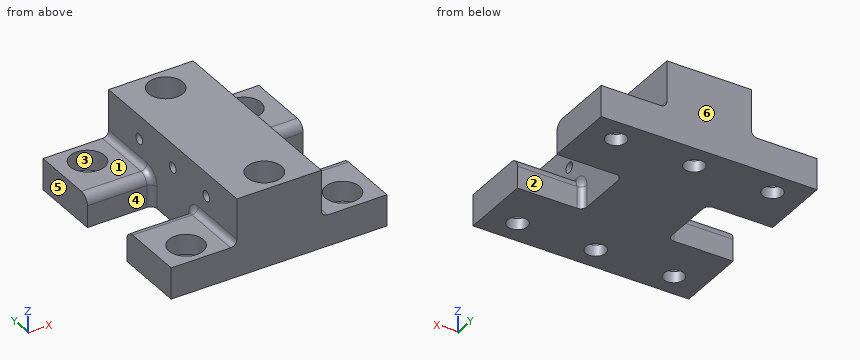
```python
from build123d import *

# Parameters (mm, degrees)
SKETCH_1_W                  = 69
SKETCH_1_H                  = 65
EXTRUDE_1_DEPTH             = 10
SKETCH_2_W                  = 27
SKETCH_2_H                  = 65
EXTRUDE_2_DEPTH             = 15
SKETCH_3_W                  = 10
SKETCH_3_H                  = 20
CUT_EXTRUDE_1_DEPTH         = 22
FILLET_1_R                  = 3
FILLET_2_R                  = 2
PATTERN_LINEAR_2_COUNT      = 2
PATTERN_LINEAR_2_PITCH      = 17
PATTERN_LINEAR_2_COL_COUNT  = 2
PATTERN_LINEAR_2_COL_PITCH  = 17
HOLE_WIZARD_M6_1_AT_2_COUNT = 2
HOLE_WIZARD_M6_1_AT_2_PITCH = 50
HOLE_WIZARD_M6_1_AT_3_COUNT = 2
HOLE_WIZARD_M6_1_AT_3_PITCH = 70.710678119
HOLE_WIZARD_M6_1_AT_4_COUNT = 2
HOLE_WIZARD_M6_1_AT_4_PITCH = 50
HOLE_WIZARD_M6_1_AT_5_COUNT = 2
HOLE_WIZARD_M6_1_AT_5_PITCH = 25
HOLE_WIZARD_M6_1_AT_6_COUNT = 2
HOLE_WIZARD_M6_1_AT_6_PITCH = 55.901699437
SKETCH_15_R                 = 5.5
CUT_EXTRUDE_3_DEPTH         = 16


with BuildPart() as part:
    # 스케치1 → 보스-돌출1 (new body)
    with BuildSketch(Plane.XY):
        Rectangle(SKETCH_1_W, SKETCH_1_H)
    extrude(amount=EXTRUDE_1_DEPTH)

    # 스케치2 → 보스-돌출2 (add)
    with BuildSketch(Plane.XY.offset(10)):
        Rectangle(SKETCH_2_W, SKETCH_2_H)
    extrude(amount=EXTRUDE_2_DEPTH)

    # 스케치3 → 컷-돌출1 (cut, through all)
    with BuildSketch(Plane(origin=(13.5, 0, 0), x_dir=(0, 0, -1), z_dir=(1, 0, 0))):
        with Locations((-5, 0)):
            Rectangle(SKETCH_3_W, SKETCH_3_H)
    cut_extrude_1 = extrude(amount=CUT_EXTRUDE_1_DEPTH, mode=Mode.SUBTRACT)

    # 대칭 복사1: 컷-돌출1 across plane
    add(cut_extrude_1.mirror(Plane(origin=(0, 0, 0), x_dir=(0, 0, 1), z_dir=(1, 0, 0))), mode=Mode.SUBTRACT)

    # 필렛1
    fillet_1_edges = [part.edges().sort_by_distance(p)[0] for p in [
        (24, 10, 10),
        (24, -10, 10),
        (-24, -10, 10),
        (-24, 10, 10),
    ]]
    fillet(fillet_1_edges, radius=FILLET_1_R)

    # 필렛2
    fillet_2_edges = [part.edges().sort_by_distance(p)[0] for p in [
        (13.5, -22.75, 10),
        (-13.5, 22.75, 10),
        (13.5, 10, 3.5),
        (-13.5, 10, 3.5),
        (-13.5, -10, 3.5),
        (-13.5, -22.75, 10),
        (13.5, -10, 3.5),
        (13.5, 22.75, 10),
        (-13.5, -10.878679656, 9.121320344),
        (-13.5, 10.878679656, 9.121320344),
        (13.5, -10.878679656, 9.121320344),
        (13.5, 10.878679656, 9.121320344),
    ]]
    fillet(fillet_2_edges, radius=FILLET_2_R)

    # 스케치8 → M4 탭을 위한 탭 드릴1 (revolve, cut)
    with BuildSketch(Plane(origin=(13.5, 0, 17.5), x_dir=(0, 0, -1), z_dir=(0, 1, 0))):
        Polygon((0, 0), (0, 7.991420021), (1.65, 7), (1.65, 0), align=None)
    hole_wizard_m4_1 = revolve(axis=Axis((19.85, 0, 17.5), (-1, 0, 0)), mode=Mode.SUBTRACT)

    # 선형 패턴2: M4 탭을 위한 탭 드릴1 ×2
    with Locations(*[(0, -i * PATTERN_LINEAR_2_PITCH, 0) for i in range(1, PATTERN_LINEAR_2_COUNT)]):
        add(hole_wizard_m4_1, mode=Mode.SUBTRACT)

    # 선형 패턴2 col: M4 탭을 위한 탭 드릴1 ×2
    with Locations(*[(0, i * PATTERN_LINEAR_2_COL_PITCH, 0) for i in range(1, PATTERN_LINEAR_2_COL_COUNT)]):
        add(hole_wizard_m4_1, mode=Mode.SUBTRACT)

    # 대칭 복사3: M4 탭을 위한 탭 드릴1 across plane
    add(hole_wizard_m4_1.mirror(Plane(origin=(0, 0, 0), x_dir=(0, 0, 1), z_dir=(1, 0, 0))), mode=Mode.SUBTRACT)

    # 대칭 복사3 copy 1 sketch → 대칭 복사3 copy 1 (revolve, cut)
    with BuildSketch(Plane(origin=(-13.5, -17, 17.5), x_dir=(0, 0, -1), z_dir=(0, 1, 0))):
        Polygon((0, 0), (0, -7.991420021), (1.65, -7), (1.65, 0), align=None)
    revolve(axis=Axis((-19.85, -17, 17.5), (-1, 0, 0)), mode=Mode.SUBTRACT)

    # 대칭 복사3 copy 2 sketch → 대칭 복사3 copy 2 (revolve, cut)
    with BuildSketch(Plane(origin=(-13.5, 17, 17.5), x_dir=(0, 0, -1), z_dir=(0, 1, 0))):
        Polygon((0, 0), (0, -7.991420021), (1.65, -7), (1.65, 0), align=None)
    revolve(axis=Axis((-19.85, 17, 17.5), (-1, 0, 0)), mode=Mode.SUBTRACT)

    # 스케치14 → M6 육각 소켓 머리 캡 나사용 카운터보어1 (revolve, cut)
    with BuildSketch(Plane(origin=(-25, 25, 10), x_dir=(0, -1, 0), z_dir=(1, 0, 0))):
        Polygon((0, 0), (0, 10), (3.2, 10), (3.2, 6.4), (5.5, 6.4), (5.5, 0), align=None)
    hole_wizard_m6_1 = revolve(axis=Axis((-25, 25, 16.35), (0, 0, -1)), mode=Mode.SUBTRACT)

    # M6 육각 소켓 머리 캡 나사용 카운터보어1 at 2: M6 육각 소켓 머리 캡 나사용 카운터보어1 ×2
    with Locations(*[(0, -i * HOLE_WIZARD_M6_1_AT_2_PITCH, 0) for i in range(1, HOLE_WIZARD_M6_1_AT_2_COUNT)]):
        add(hole_wizard_m6_1, mode=Mode.SUBTRACT)

    # M6 육각 소켓 머리 캡 나사용 카운터보어1 at 3: M6 육각 소켓 머리 캡 나사용 카운터보어1 ×2
    with Locations(*[Vector(0.707106781, -0.707106781, 0) * (i * HOLE_WIZARD_M6_1_AT_3_PITCH) for i in range(1, HOLE_WIZARD_M6_1_AT_3_COUNT)]):
        add(hole_wizard_m6_1, mode=Mode.SUBTRACT)

    # M6 육각 소켓 머리 캡 나사용 카운터보어1 at 4: M6 육각 소켓 머리 캡 나사용 카운터보어1 ×2
    with Locations(*[(i * HOLE_WIZARD_M6_1_AT_4_PITCH, 0, 0) for i in range(1, HOLE_WIZARD_M6_1_AT_4_COUNT)]):
        add(hole_wizard_m6_1, mode=Mode.SUBTRACT)

    # M6 육각 소켓 머리 캡 나사용 카운터보어1 at 5: M6 육각 소켓 머리 캡 나사용 카운터보어1 ×2
    with Locations(*[(i * HOLE_WIZARD_M6_1_AT_5_PITCH, 0, 0) for i in range(1, HOLE_WIZARD_M6_1_AT_5_COUNT)]):
        add(hole_wizard_m6_1, mode=Mode.SUBTRACT)

    # M6 육각 소켓 머리 캡 나사용 카운터보어1 at 6: M6 육각 소켓 머리 캡 나사용 카운터보어1 ×2
    with Locations(*[Vector(0.447213595, -0.894427191, 0) * (i * HOLE_WIZARD_M6_1_AT_6_PITCH) for i in range(1, HOLE_WIZARD_M6_1_AT_6_COUNT)]):
        add(hole_wizard_m6_1, mode=Mode.SUBTRACT)

    # 스케치15 → 컷-돌출3 (cut, through all)
    with BuildSketch(Plane(origin=(0, 0, 10), x_dir=(-1, 0, 0), z_dir=(0, 0, -1))):
        with Locations((0, -25)):
            Circle(SKETCH_15_R)
        with Locations((0, 25)):
            Circle(SKETCH_15_R)
    extrude(amount=-CUT_EXTRUDE_3_DEPTH, mode=Mode.SUBTRACT)


solid = part.part
```
Check sheet for the modelled part. Datum: model origin and axes. Units: mm. Face numbers are marked on the shaded views. A direction names the side the tool comes from. Round coordinates to 2 decimals unless told otherwise and drop trailing zeros. Loops run counter-clockwise (first coordinate to the right, second up) from the corner with the lowest first, then second, coordinate; pieces in that order, holes last. Notation, with made-up numbers: M 37.5,-36 L 91.5,-36 A9 ccw 91.5,-26 Z; hole C -31,73 d6. An arc over 180 degrees is marked long. Answer as a JSON object with one key per item and string values.
1. Section check B-B (x = 1.5). Record the boundary of the cut face in (y, z).
Reply:
{"outline": "M -32.5,0 L -27.83,0 L -27.83,3.6 L -30.29,3.6 L -30.29,25 L -32.5,25 Z; M -22.17,0 L 22.17,0 L 22.17,3.6 L 19.71,3.6 L 19.71,25 L -19.71,25 L -19.71,3.6 L -22.17,3.6 Z; M 27.83,0 L 32.5,0 L 32.5,25 L 30.29,25 L 30.29,3.6 L 27.83,3.6 Z"}
2. Access from +Z, -Z, +X, -X, +Y, -Y to the whole of each face (thin tool, end or side, straight path). Record for the marked faces 1, 2 and 3.
Reply:
{"face 1": "+Z, -X, +Y, -Y", "face 2": "+Z, -Z, +X", "face 3": "+Z"}
3. Scan lines: line 1 (X direction, y = 25, z = 2.1); line 2 (Y direction, x = -25, z = 2.8); line 3 (Y direction, x = 0, z = 1.05). Record each from-to range of solid material in increasing order.
Reply:
{"line 1": "x = -34.5 to -28.2, -21.8 to -3.2, 3.2 to 21.8, 28.2 to 34.5", "line 2": "y = -32.5 to -28.2, -21.8 to -10, 10 to 21.8, 28.2 to 32.5", "line 3": "y = -32.5 to -28.2, -21.8 to 21.8, 28.2 to 32.5"}
4. Section check D-D (y = -14). Record the boundary of the cut face in (x, z), plus the area to 3 significant figures.
Reply:
{"outline": "M -34.5,0 L 34.5,0 L 34.5,10 L 15.5,10 A2 cw 13.5,12 L 13.5,25 L -13.5,25 L -13.5,12 A2 cw -15.5,10 L -34.5,10 Z", "area": "1,100 mm²"}
5. Section check A-A (z = 6). Record the boundary of the cut face in (x, y), plus the area to 3 significant figures.
Reply:
{"outline": "M -34.5,-32.5 L 34.5,-32.5 L 34.5,-10 L 15.5,-10 A2 cw 13.5,-8 L 13.5,8 A2 cw 15.5,10 L 34.5,10 L 34.5,32.5 L -34.5,32.5 L -34.5,10 L -15.5,10 A2 cw -13.5,8 L -13.5,-8 A2 cw -15.5,-10 L -34.5,-10 Z; hole C -25,-25 d11; hole C -25,25 d11; hole C 0,-25 d11; hole C 0,25 d11; hole C 25,-25 d11; hole C 25,25 d11", "area": "3,080 mm²"}
6. Gauge pin test, flat ends, axial feed: P1, Ø10, axis at x = 0, y = -25, coming from the +Z side; P2, Ø2, axis at y = 2, z = 16.5, coming from the +X side; P3, Ø10, axis at x = 0, y = 25, coming from the -Z side; P4, Ø2, axis at y = -7.5, z = 3.5, coming from the -X side. Record the tip position at first contact, or that the pin passes through.
Reply:
{"P1": "stops at z = 3.6", "P2": "stops at x = 13.5", "P3": "stops at z = 0", "P4": "stops at x = -13.56"}
7. Section check C-C (x = 29). Record the boundary of the cut face in (y, z).
Reply:
{"outline": "M -32.5,0 L -10,0 L -10,7 A3 ccw -13,10 L -21.23,10 L -21.23,3.6 L -28.77,3.6 L -28.77,10 L -32.5,10 Z; M 10,0 L 32.5,0 L 32.5,10 L 28.77,10 L 28.77,3.6 L 21.23,3.6 L 21.23,10 L 13,10 A3 ccw 10,7 Z"}
8. Mould release check, pull along Y, two halves, no side actions. Record for the marked faces 4, 5 and 6: pulls with the +Y half, pulls with the -Y half, needs draft (parallel to the pull), parting line crosses it, or undercut.
Reply:
{"face 4": "undercut", "face 5": "needs draft", "face 6": "pulls with the +Y half"}
